```python
from build123d import *

# Parameters (mm, degrees)
SKETCH1_W                = 9.5
SKETCH1_H                = 54.75
BOSS_EXTRUDE1_DEPTH      = 9.5
SKETCH2_R                = 7.5
BOSS_EXTRUDE2_DEPTH      = 19
BOSS_EXTRUDE2_DEPTH_BACK = 9.5
BOSS_EXTRUDE3_DEPTH      = 8


with BuildPart() as part:
    # Sketch1 → Boss-Extrude1 (new body)
    with BuildSketch(Plane(origin=(0, 0, 0), x_dir=(1, 0, 0), z_dir=(0, 1, 0))):
        Rectangle(SKETCH1_W, SKETCH1_H)
    extrude(amount=BOSS_EXTRUDE1_DEPTH)

    # Sketch2 → Boss-Extrude2 (add, two sides)
    with BuildSketch(Plane(origin=(0, 9.5, 0), x_dir=(1, 0, 0), z_dir=(0, 1, 0))) as boss_extrude2_sk:
        with Locations((0, -27.375)):
            Circle(SKETCH2_R)
    extrude(amount=BOSS_EXTRUDE2_DEPTH)
    extrude(boss_extrude2_sk.sketch, amount=-BOSS_EXTRUDE2_DEPTH_BACK)

    # Sketch3 → Boss-Extrude3 (add)
    with BuildSketch(Plane(origin=(0, 28.5, 0), x_dir=(1, 0, 0), z_dir=(0, 1, 0))):
        with BuildLine():
            Line((-1.29624151, -30.947080339), (-1.29624151, -27.289433429))
            Line((-1.29624151, -27.289433429), (-3.391270856, -27.289433429))
            Line((-3.391270856, -27.289433429), (-3.391270856, -29.089433429))
            ThreePointArc((-3.391270856, -29.089433429), (1.102654775, -23.738497223), (1.86802767, -30.684149834))
            Line((1.86802767, -30.684149834), (0.894110574, -30.684149834))
            Line((0.894110574, -30.684149834), (0.894110574, -31.065442297))
            Line((0.894110574, -31.065442297), (-0.905889426, -31.065442297))
            ThreePointArc((-0.905889426, -31.065442297), (-1.102654775, -31.011502777), (-1.29624151, -30.947080339))
        make_face()
    extrude(amount=BOSS_EXTRUDE3_DEPTH)


solid = part.part
```
The listing builds one solid part. Answer for the finished solid, in the listing's coordinates (mm). A direction names the side the tool comes from. Give positions to 0.01 mm unless a question says otherwise; leave off trailing zeros. Loops run counter-clockwise (first coordinate to the right, second up) from the corner with the lowest first, then second, coordinate; pieces in that order, holes last. Notation, with made-up numbers: (72, 24.5) - (99, 24.5) arc R18 ccw to (99, 39.5) - close; hole circle Ø10 at (59, -17.75). An arc over 180 degrees is marked (long way). Return JSON: item names as keys, results as strings. Group by question number.
1. Find section D-D (y = 23). Write down the section's boundary in (x, z) (3 decimals).
2. Which of the six approach directions +Z, -Z, +X, -X, +Y, -Y give full straight-line access (tool end or side, diameter ignored) to faces 1 (the flat face through (0, 5, -27.375)), 2 (the flat face through (-4.75, 5, -3)), 3 (the flat face through (-3.391, 32, 28)), 4 (the cylindrical face through (0.983, 32.444, 23.704))?
3. Given pin 1 Ø0.8 at (x, y) = (1, 34) entering from +Z; pin 2 Ø1 at (x, y) = (5.5, 22.5) entering from +Z; pin 3 Ø6 at (x, y) = (-6, 22) entering from +Z, each flat-ended and moving along its own axis, determine where each tip first touches the part or whether it passes through.
4. Find section A-A (x = 0). Write down the section's boundary in (y, z) (3 decimals), then the cut area to 3 significant figures.
5. Find section B-B (y = 29.5). Write down the section's boundary in (x, z) (3 decimals), then the cut area to 3 significant figures.
6. Determine the mould class of faces 5 (the flat face through (-2, 32, 27.289)), 6 (the flat face through (4.75, 5, -3)), 7 (the flat face through (0, 32, 31.065)) for opening direction X: pulls with the +X half, pulls with the -X half, needs draft (parallel to the pull), parting line crosses it, or undercut.
7. Straight lines are drawn through the part: line 1 (Y direction, x = 4, z = 13); line 2 (X direction, y = 4.5, z = -18); line 3 (Z direction, x = -0.25, y = 9) (3 decimals). For each, find the intervals that lie inside material, in ascending order. Write a range as [from, to].
8. Find section C-C (z = -22). Write down the section's boundary in (x, y).
Verdict:
{
 "1": {"outline": "circle Ø15 at (0, 27.375)"},
 "2": {"face 1": "-Z, +X, -X, +Y, -Y", "face 2": "-Z, -X, +Y, -Y", "face 3": "+Z, +Y", "face 4": "+Y"},
 "3": {"pin 1": "stops at z = 31.07", "pin 2": "stops at z = 32.97", "pin 3": "stops at z = 34.25"},
 "4": {"outline": "(0, -27.375) - (9.5, -27.375) - (9.5, 19.875) - (28.5, 19.875) - (28.5, 23.575) - (36.5, 23.575) - (36.5, 31.065) - (28.5, 31.065) - (28.5, 34.875) - (0, 34.875) - close", "area": "936 mm^2"},
 "5": {"outline": "(-3.391, 27.289) - (-3.391, 29.089) arc R3.8 ccw (long way) to (1.868, 30.684) - (0.894, 30.684) - (0.894, 31.065) - (-0.906, 31.065) arc R3.8 ccw to (-1.296, 30.947) - (-1.296, 27.289) - close", "area": "38.8 mm^2"},
 "6": {"face 5": "undercut", "face 6": "pulls with the +X half", "face 7": "needs draft"},
 "7": {"line 1": "y = [0, 9.5]", "line 2": "x = [-4.75, 4.75]", "line 3": "z = [-27.375, 34.871]"},
 "8": {"outline": "(-4.75, 0) - (4.75, 0) - (4.75, 9.5) - (-4.75, 9.5) - close"}
}
